Print and shaded views of the part. All mm, measured from the part's lowest x, y and z. A direction names the side the tool comes from. Round coordinates to 2 decimals unless told otherwise and drop trailing zeros. Write each loop counter-clockwise with the first axis right and the second up, starting at its lowest first coordinate (ties: lowest second). Pieces come first, ordered by that corner, then holes.
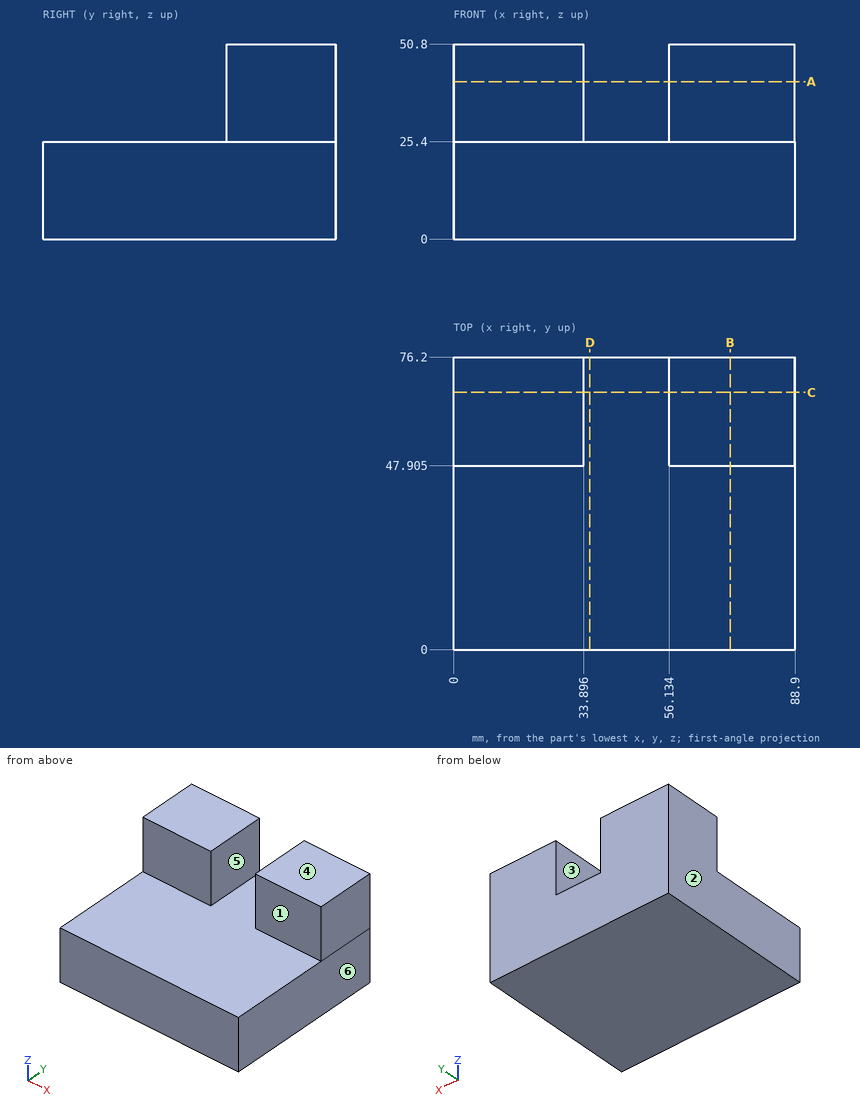
1) Which spindle directions (+Z, -Z, +X, -X, +Y, -Y) get a long thin tool onto all of the face, cutting with end or side? Do the marked faces 1, 2 and 3. Say none if no direction does.
Results:
face 1: +Z, +X, -X, -Y
face 2: +Z, -Z, -X, +Y, -Y
face 3: +Z, +Y, -Y
2) Slice it at D-D (x = 35.5). Write the cut outline in (y, z).
Results:
outline: (0, 0) - (76.2, 0) - (76.2, 25.4) - (0, 25.4) - close
3) Slice it at B-B (x = 72). Write the cut outline in (y, z) (1 decimal), plus the area to 3 significant figures.
Results:
outline: (0, 0) - (76.2, 0) - (76.2, 50.8) - (47.9, 50.8) - (47.9, 25.4) - (0, 25.4) - close
area: 2,650 mm2
4) Slice it at C-C (y = 67). Write the cut outline in (x, z), plus the area to 3 significant figures.
Results:
outline: (0, 0) - (88.9, 0) - (88.9, 50.8) - (56.13, 50.8) - (56.13, 25.4) - (33.9, 25.4) - (33.9, 50.8) - (0, 50.8) - close
area: 3,950 mm2
5) Pin check, flat tips, straight feed: pin 1 Ø12 at (x, y) = (52.5, 33.5) entering from +Z; pin 2 Ø12 at (x, z) = (64.5, 17.5) entering from -Y; pin 3 Ø1 at (x, z) = (60, 39.5) entering from -Y (1 decimal). Stop position of each tip, or through.
Results:
pin 1: stops at z = 25.4
pin 2: stops at y = 0
pin 3: stops at y = 47.9
6) Slice it at A-A (z = 41). Write the cut outline in (x, y) (1 decimal).
Results:
outline: (0, 47.9) - (33.9, 47.9) - (33.9, 76.2) - (0, 76.2) - close; (56.1, 47.9) - (88.9, 47.9) - (88.9, 76.2) - (56.1, 76.2) - close
7) Wall check: L1, parallel to X at y = 48.5, z = 31.5; L2, parallel to Z at x = 36, y = 47; L3, parallel to Y at x = 32.5, z = 27 (1 decimal). Give the ranges that are in metal, low to high.
Results:
L1: x = 0 to 33.9, 56.13 to 88.9
L2: z = 0 to 25.4
L3: y = 47.9 to 76.2
8) Mould opens along X. For the marked faces 4, 5 and 6 say: released by +X, released by -X, zero draft, split by the parting line, or undercut.
Results:
face 4: zero draft
face 5: undercut
face 6: released by +X
